Autodesk Inventor part; units mm, degrees
ref_plane "YZ Plane" through (0, 0, 0) normal (1, 0, 0) x (0, 1, 0)
ref_plane "XZ Plane" through (0, 0, 0) normal (0, 1, 0) x (-1, 0, 0)
ref_plane "XY Plane" through (0, 0, 0) normal (0, 0, 1) x (1, 0, 0)
sketch "Sketch1" plane through (0, 0, 0) normal (0, 0, 1) x (1, 0, 0)
  line L0 (-44.7811, 27.3777) -> (-44.7811, 21.678)
  line L1 (69.7802, 27.3777) -> (69.7802, 21.678)
  line L2 (69.7802, 27.3777) -> (69.7802, 21.678)
  line L3 (-44.7811, 21.678) -> (-31.9793, 21.678)
  line L4 (-31.9793, 27.3777) -> (-31.9793, 21.678)
  line L5 (-31.9793, 27.3777) -> (-31.9793, 21.678)
  line L6 (-20.8402, 21.678) -> (-20.8402, 27.3777)
  line L7 (-20.8402, 27.3777) -> (-20.8402, 21.678)
  line L8 (4.7205, 21.678) -> (4.7205, 27.3777)
  line L9 (4.7205, 27.3777) -> (4.7205, 21.678)
  line L10 (20.2786, 27.3777) -> (20.2786, 21.678)
  line L11 (20.2786, 27.3777) -> (20.2786, 21.678)
  line L12 (31.9768, 27.3777) -> (31.9768, 21.678)
  line L13 (45.8394, 27.3777) -> (45.8394, 21.678)
  line L14 (45.8394, 27.3777) -> (45.8394, 21.678)
  line L15 (56.9784, 21.678) -> (69.7802, 21.678)
  line L16 (56.9784, 27.3777) -> (56.9784, 21.678)
  line L17 (-6.9776, 27.3777) -> (-6.9776, 21.678)
  line L18 (-31.9793, 21.678) -> (-44.7811, 21.678)
  line L19 (-6.9776, 21.678) -> (-20.8402, 21.678)
  line L20 (20.2786, 21.678) -> (4.7205, 21.678)
  line L21 (69.7802, 21.678) -> (56.9784, 21.678)
  line L22 (45.8394, 21.678) -> (31.9768, 21.678)
  line L23 (-44.7811, 27.3777) -> (-44.7811, 83.2577)
  line L24 (-44.7811, 83.2577) -> (69.7802, 83.2577)
  line L25 (69.7802, 83.2577) -> (69.7802, 27.3777)
  line L26 (56.9784, 27.3777) -> (45.8394, 27.3777)
  line L27 (31.9768, 27.3777) -> (20.2786, 27.3777)
  line L28 (4.7205, 27.3777) -> (-6.9776, 27.3777)
  line L29 (-20.8402, 27.3777) -> (-31.9793, 27.3777)
  point P0 (0, 0)
  dimension "d0" = 55.88
extrude "Extrusion1" add sketch "Sketch1" along normal blind 2.286
sketch "Sketch2" plane through (0, 0, 2.286) normal (0, 0, 1) x (1, 0, 0)
  line L0 (-31.9793, 21.678) -> (-31.9793, 27.3777)
  line L1 (-44.7811, 83.2577) -> (-44.7811, 21.678)
  line L2 (-44.7811, 27.3777) -> (-46.3559, 27.3777)
  line L3 (-44.7811, 83.2577) -> (-46.3559, 83.2577)
  line L4 (-46.3559, 83.2577) -> (-46.3559, 27.3777)
  line L5 (69.7802, 83.2577) -> (-44.7811, 83.2577)
  line L6 (69.7802, 27.3777) -> (71.355, 27.3777)
  line L7 (71.355, 83.2577) -> (71.355, 27.3777)
  line L8 (-44.7811, 83.2577) -> (-44.7811, 27.3777)
  line L9 (69.7802, 83.2577) -> (71.355, 83.2577)
  line L10 (69.7802, 21.678) -> (69.7802, 83.2577)
  line L11 (69.7802, 83.2577) -> (69.7802, 27.3777)
  point P0 (0, 0)
  dimension "d3" = 1.5748
extrude "Extrusion2" add sketch "Sketch2" against normal blind 2.286
sketch "Sketch3" plane through (0, 0, 2.286) normal (0, 0, 1) x (1, 0, 0)
  point P0 (0, 0)
properties part number "mcdave_ramp"
Read the model definition and answer for the solid it produces. Units are mm, in the model's axes. A direction names the side the tool comes from. Coordinates: 2 decimals unless noted, no trailing zeros. Write each loop counter-clockwise with the first axis right and the second up, starting at its lowest first coordinate (ties: lowest second). Pieces come first, ordered by that corner, then holes. Notation, with made-up numbers: M 36.5,-33.5 L 53.5,-33.5 A20 ccw 53.5,-2.5 Z; hole C 4.25,-32.75 d11. An arc over 180 degrees is marked long. Use a Markdown table: item, result.
Q1. The part is cut by section B-B, the plane x = 55. Write down the section's boundary in (y, z).
Answer block:
| item | result |
|---|---|
| outline | M 27.38,0 L 83.26,0 L 83.26,2.29 L 27.38,2.29 Z |
Q2. Which of the six approach directions +Z, -Z, +X, -X, +Y, -Y give full straight-line access (tool end or side, diameter ignored) to faces 1 (the face through (-44.781, 25, 1)), 2 (the face through (45.839, 25, 1)), 3 (the face through (69.78, 25, 1))?
Answer block:
| item | result |
|---|---|
| face 1 | +Z, -Z, -X, -Y |
| face 2 | +Z, -Z, -Y |
| face 3 | +Z, -Z, +X, -Y |
Q3. The part is cut by section A-A, the plane z = 0.85. Write down the section's boundary in (x, y) (1 decimal).
Answer block:
| item | result |
|---|---|
| outline | M -46.4,27.4 L -44.8,27.4 L -44.8,21.7 L -32,21.7 L -32,27.4 L -20.8,27.4 L -20.8,21.7 L -7,21.7 L -7,27.4 L 4.7,27.4 L 4.7,21.7 L 20.3,21.7 L 20.3,27.4 L 32,27.4 L 32,21.7 L 45.8,21.7 L 45.8,27.4 L 57,27.4 L 57,21.7 L 69.8,21.7 L 69.8,27.4 L 71.4,27.4 L 71.4,83.3 L -46.4,83.3 Z |
Q4. Determine the mould class of faces 4 (the face through (12, 53, 0)), 5 (the face through (-31.979, 25, 1)), 6 (the face through (-46.356, 56, 1)), 7 (the face through (-20.84, 24, 1)) for opening direction X: released by +X, released by -X, zero draft, split by the parting line, or undercut.
Answer block:
| item | result |
|---|---|
| face 4 | zero draft |
| face 5 | undercut |
| face 6 | released by -X |
| face 7 | undercut |
Q5. A straight line is drawn through the part: L1, parallel to Y at x = 28, z = 0.95. Find the intervals that lie inside material, in ascending order. Write a range as [from, to].
Answer block:
| item | result |
|---|---|
| L1 | y = [27.38, 83.26] |
Q6. Each of these flat-tipped pins is pushed along its axis until it touches: pin 1 Ø2 at (x, y) = (6.5, 71) entering from -Z; pin 2 Ø0.7 at (y, z) = (25.5, 1.5) entering from +X; pin 3 Ø1.1 at (x, z) = (53.5, 1) entering from -Y; pin 4 Ø1.1 at (y, z) = (26, 0.5) entering from -X. Where does it stop, or does it pass through?
Answer block:
| item | result |
|---|---|
| pin 1 | stops at z = 0 |
| pin 2 | stops at x = 69.78 |
| pin 3 | stops at y = 27.38 |
| pin 4 | stops at x = -44.78 |
